from build123d import *

# Parameters (mm, degrees)
CROQUIS1_R                 = 8
SALIENTE_EXTRUIR1_DEPTH    = 11
CROQUIS2_W                 = 11
CROQUIS2_H                 = 16
SALIENTE_EXTRUIR2_DEPTH    = 16
CROQUIS3_R                 = 5.1
CORTAR_EXTRUIR1_DEPTH      = 20
CORTAR_EXTRUIR2_DEPTH      = 22
CORTAR_EXTRUIR2_DEPTH_BACK = 22
CROQUIS4_R                 = 4.15
REDONDEO2_R                = 1
REDONDEO3_R                = 1


with BuildPart() as part:
    # Croquis1 → Saliente-Extruir1 (new body)
    with BuildSketch(Plane.XY):
        Circle(CROQUIS1_R)
    extrude(amount=SALIENTE_EXTRUIR1_DEPTH)

    # Croquis2 → Saliente-Extruir2 (add)
    with BuildSketch(Plane(origin=(0, 0, 0), x_dir=(0, 0, -1), z_dir=(1, 0, 0))):
        with Locations((-5.5, 0)):
            Rectangle(CROQUIS2_W, CROQUIS2_H)
    extrude(amount=SALIENTE_EXTRUIR2_DEPTH)

    # Croquis3 → Cortar-Extruir1 (cut)
    with BuildSketch(Plane.XY.offset(11)):
        Circle(CROQUIS3_R)
    extrude(amount=-CORTAR_EXTRUIR1_DEPTH, mode=Mode.SUBTRACT)

    # Croquis4 → Cortar-Extruir2 (cut, two sides: drawn at the far end of the back side and taken through both)
    with BuildSketch(Plane(origin=(0, 0, 0), x_dir=(1, 0, 0), z_dir=(0, 1, 0)).offset(-CORTAR_EXTRUIR2_DEPTH_BACK)):
        with Locations(Location((11, -5.5, 0), (0, 0, 270))):
            Circle(CROQUIS4_R)
    extrude(amount=CORTAR_EXTRUIR2_DEPTH + CORTAR_EXTRUIR2_DEPTH_BACK, mode=Mode.SUBTRACT)

    # Redondeo2
    redondeo2_edges = [part.edges().sort_by_distance(p)[0] for p in [
        (16, 0, 0),
    ]]
    fillet(redondeo2_edges, radius=REDONDEO2_R)

    # Redondeo3
    redondeo3_edges = [part.edges().sort_by_distance(p)[0] for p in [
        (16, 0, 11),
    ]]
    fillet(redondeo3_edges, radius=REDONDEO3_R)


solid = part.part
Source: CAD feature listing. Evaluate the final solid. Frame: model axes, mm. Give positions to 0.01 mm unless a question says otherwise; leave off trailing zeros. Loops run counter-clockwise (first coordinate to the right, second up) from the corner with the lowest first, then second, coordinate; pieces in that order, holes last. Notation, with made-up numbers: (-36, 86) -> (-6, 86) arc R17 ccw to (-6, 110) -> close; hole circle Ø5 at (70, -30.75). An arc over 180 degrees is marked (long way). Use a Markdown table: item, result. Add a question column.
1) Section query A-A, the plane y = 0. Return the cut outline in (x, z), then the cut area to 3 significant figures.
2) Pull-direction query (X, two-part tool) for faces 1 (the face through (15.715, 0.112, 0.301)), 2 (the face through (6, 0, 11)), 3 (the face through (6.95, -0.11, 4.6)), 4 (the face through (2.4, -4.5, 5.6)); classes: +X half, -X half, draft (parallel to the pull), parting line (faces both ways), or undercut.
3) Section query D-D, the plane y = 7.25. Return the cut outline in (x, z).
4) Section query B-B, the plane z = 4.5. Return the cut outline in (x, y).
5) Line query: line 1 along Z through (x, y) = (11, 4); line 2 along X through (y, z) = (-1.5, 6); line 3 along X through (y, z) = (2.5, 6.5). Output: solid intervals per line, ascending. Write a range as [from, to].
6) Section query C-C, the plane x = 11. Return the cut outline in (y, z).
7) First-contact query: pin 1 (3 mm diameter, centred on y = -3, z = 8.5, fed in from -X); pin 2 (2 mm diameter, centred on x = 1.5, y = 3.5, fed in from -Z); pin 3 (2 mm diameter, centred on x = 7.5, z = 5, fed in from -Y); pin 4 (1 mm diameter, centred on y = -2.5, z = 2, fed in from -X). Flat tips, straight axial feed; report the tip coordinate or a pass-through.
Numbers:
| question | item | result |
|---|---|---|
| 1 | outline | (-8, 0) -> (-5.1, 0) -> (-5.1, 11) -> (-8, 11) -> close; (5.1, 0) -> (15, 0) arc R1 ccw to (16, 1) -> (16, 10) arc R1 ccw to (15, 11) -> (5.1, 11) -> close; hole circle Ø8.3 at (11, 5.5) |
| 1 | area | 97.3 mm2 |
| 2 | face 1 | +X half |
| 2 | face 2 | draft |
| 2 | face 3 | undercut |
| 2 | face 4 | undercut |
| 3 | outline | (-3.38, 0) -> (15, 0) arc R1 ccw to (16, 1) -> (16, 10) arc R1 ccw to (15, 11) -> (-3.38, 11) -> close; hole circle Ø8.3 at (11, 5.5) |
| 4 | outline | (0, -8) -> (6.97, -8) -> (6.97, 8) -> (0, 8) arc R8 ccw to start; (15.03, -8) -> (16, -8) -> (16, 8) -> (15.03, 8) -> close; hole circle Ø10.2 at (0, 0) |
| 5 | line 1 | z = [0, 1.35], [9.65, 11] |
| 5 | line 2 | x = [-7.86, -4.87], [4.87, 6.88], [15.12, 16] |
| 5 | line 3 | x = [-7.6, -4.45], [4.45, 6.97], [15.03, 16] |
| 6 | outline | (-8, 0) -> (8, 0) -> (8, 1.35) -> (-8, 1.35) -> close; (-8, 9.65) -> (8, 9.65) -> (8, 11) -> (-8, 11) -> close |
| 7 | pin 1 | stops at x = -7.86 |
| 7 | pin 2 | passes through |
| 7 | pin 3 | stops at y = -8 |
| 7 | pin 4 | stops at x = -7.75 |
